Geometry: final body of the model. Coordinates: model frame, mm. A direction names the side the tool comes from. Coordinates: 2 decimals unless noted, no trailing zeros. Loops run counter-clockwise (first coordinate to the right, second up) from the corner with the lowest first, then second, coordinate; pieces in that order, holes last. Notation, with made-up numbers: (65.5, 59) - (76.5, 59) arc R26 ccw to (76.5, 98) - close; hole circle Ø11 at (86, 1). An arc over 180 degrees is marked (long way). Return JSON: item names as keys, results as strings.
from build123d import *


with BuildPart() as part:
    # Çizim1 → Döndür1 (revolve)
    with BuildSketch(Plane.XY, mode=Mode.PRIVATE) as d_nd_r1_sk:
        Polygon((-5.608586602, 3.125), (9.391413398, 3.125), (9.391413398, 5), (4.391413398, 5), (4.391413398, 16.5), (9.391413398, 16.5), (9.391413398, 20), (5.391413398, 20), (1.891413398, 18.256578947), (-1.608586602, 20), (-5.608586602, 20), (-5.608586602, 16.5), (-0.608586602, 16.5), (-0.608586602, 5), (-5.608586602, 5), align=None)
    revolve(d_nd_r1_sk.sketch.rotate(Axis((-7.63862782, 0, 0), (1, 0, 0)), 90), axis=Axis((-7.63862782, 0, 0), (1, 0, 0)))


solid = part.part
Item 1: Ray query, probe 1 along Y at (x, z) = (-2, 0) (3 decimals); probe 2 along Z at (x, y) = (-4.25, -2); probe 3 along X at (y, z) = (13.5, -9). Return the intervals inside material, ascending. Write a range as from..to.
Worked out:
{"probe 1": "-20..-16.5, -5..-3.125, 3.125..5, 16.5..20", "probe 2": "-19.9..-16.38, -4.58..-2.4, 2.4..4.58, 16.38..19.9", "probe 3": "-0.61..4.39"}
Item 2: Section query A-A, the plane x = -2.5. Return loops of the section in (y, z) (3 decimals), and give its area (3 significant figures).
Worked out:
{"outline": "circle Ø40 at (0, 0); circle Ø10 at (0, 0); hole circle Ø33 at (0, 0); hole circle Ø6.25 at (0, 0)", "area": "449 mm^2"}
Item 3: First-contact query: pin 1 Ø10 at (y, z) = (7, -7.5) entering from +X; pin 2 Ø4 at (x, z) = (7.5, 15.5) entering from -Y; pin 3 Ø4 at (x, y) = (3.5, 10.5) entering from -Z. Flat tips, straight axial feed; report the tip coordinate or a pass-through.
Worked out:
{"pin 1": "x = 4.39", "pin 2": "y = -14.76", "pin 3": "z = -17.55"}
Item 4: Reachability of faces 1 (the face through (-0.609, 3.4, -3.9)), 2 (the face through (-3.64, -0.88, -19.98)), 3 (the face through (2.061, -5.509, 17.494)), 4 (the face through (6.926, -4.956, 15.738)) from +Z, -Z, +X, -X, +Y, -Y: full face, straight path, thin tool, end or side. Return the list, or none.
Worked out:
{"face 1": "-X", "face 2": "+X, -X", "face 3": "none", "face 4": "+X"}
Item 5: Mould query, pull axis Y, two halves, no side actions, for faces 5 (the face through (2, -0.94, 2.98)), 6 (the face through (7.36, -0.88, -19.98)), 7 (the face through (9.391, -16.4, -2.9)). Classes: +Y half, -Y half, draft (parallel to the pull), parting line (faces both ways), or undercut.
Worked out:
{"face 5": "undercut", "face 6": "parting line", "face 7": "draft"}
